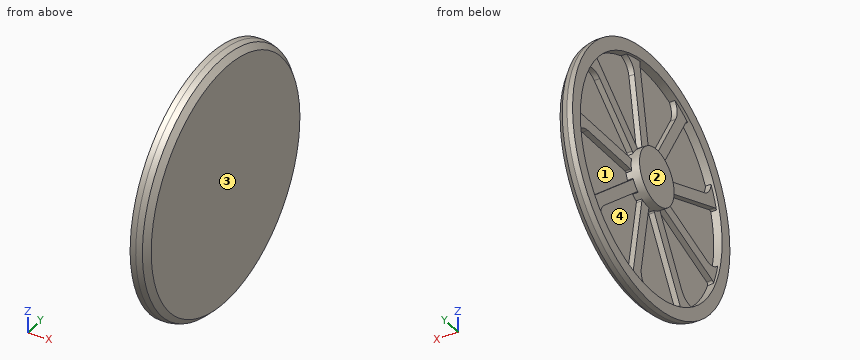
```python
from build123d import *

# Parameters (mm, degrees)
BOSS_EXTRU_1_DEPTH           = 20
R_P_TITION_CIRCULAIRE1_COUNT = 9


with BuildPart() as part:
    # Esquisse1 → Révolution1 (revolve)
    with BuildSketch(Plane.XY, mode=Mode.PRIVATE) as r_volution1_sk:
        Polygon((0, 0), (0, 430), (-19.509618943, 449.509618943), (-40, 455), (-60, 455), (-60, 410), (-30, 410), (-30, 100), (-80, 100), (-80, 0), align=None)
    revolve(r_volution1_sk.sketch.rotate(Axis((-80, 0, 0), (1, 0, 0)), 90), axis=Axis((-80, 0, 0), (1, 0, 0)))

    # Esquisse2 → Boss.-Extru.1 (add)
    with BuildSketch(Plane.ZY.offset(30)):
        with BuildLine():
            Line((-20, 104.612235173), (-20, 350.590090575))
            ThreePointArc((-20, 350.590090575), (-30.106477192, 383.916302208), (-57.021212726, 406.015493915))
            ThreePointArc((-57.021212726, 406.015493915), (-15.546179109, 409.705157784), (26.089198597, 409.169101615))
            ThreePointArc((26.089198597, 409.169101615), (21.660095503, 405.483324106), (20, 399.965535329))
            Line((20, 399.965535329), (20, 103.482062221))
            ThreePointArc((20, 103.482062221), (20.497231695, 100.367998231), (21.939478907, 97.563616504))
            ThreePointArc((21.939478907, 97.563616504), (-0.653338085, 99.997865724), (-23.212419248, 97.268615661))
            ThreePointArc((-23.212419248, 97.268615661), (-20.838236864, 100.60448066), (-20, 104.612235173))
        make_face()
    boss_extru_1 = extrude(amount=BOSS_EXTRU_1_DEPTH)

    # Répétition circulaire1: Boss.-Extru.1 ×9 about axis
    r_p_tition_circulaire1_axis = Axis((0, 0, 0), (1, 0, 0))
    for i in range(1, R_P_TITION_CIRCULAIRE1_COUNT):
        add(boss_extru_1.rotate(r_p_tition_circulaire1_axis, i * 360 / R_P_TITION_CIRCULAIRE1_COUNT))


solid = part.part
```
Verification items for the finished model (mm, model axes). Face numbers are marked on the shaded views. A direction names the side the tool comes from. Coordinates: 2 decimals unless noted, no trailing zeros. Write each loop counter-clockwise with the first axis right and the second up, starting at its lowest first coordinate (ties: lowest second). Pieces come first, ordered by that corner, then holes. Notation, with made-up numbers: M 45.25,41 L 87.25,41 A16 cw 87.25,71 Z; hole C 61,35 d4. An arc over 180 degrees is marked long. One line per item, written item: value.
Item 1: Mould release check, pull along Y, two halves, no side actions. Record for the marked faces 1 and 2: pulls with the +Y half, pulls with the -Y half, needs draft (parallel to the pull), parting line crosses it, or undercut.
Check sheet entries:
face 1: undercut
face 2: needs draft
Item 2: Section check A-A, the plane z = 0. Record the boundary of the cut face in (x, y).
Check sheet entries:
outline: M -80,-100 L -30,-100 L -30,-410 L -60,-410 L -60,-455 L -40,-455 L -19.51,-449.51 L 0,-430 L 0,430 L -19.51,449.51 L -40,455 L -60,455 L -60,410 L -50,410 L -50,100 L -80,100 Z
Item 3: Access from +Z, -Z, +X, -X, +Y, -Y to the whole of each face (thin tool, end or side, straight path). Record for the marked faces 3 and 4.
Check sheet entries:
face 3: +Z, -Z, +X, +Y, -Y
face 4: -X
Item 4: Gauge pin test, flat ends, axial feed: pin 1 Ø8 at (x, z) = (-63.5, -209.5) entering from +Y; pin 2 Ø10 at (x, z) = (-66.5, 97) entering from -Y; pin 3 Ø16 at (x, y) = (-41.5, 256.5) entering from -Z. Record the tip position at first contact, or that the pin passes through.
Check sheet entries:
pin 1: stops at y = 404.9
pin 2: stops at y = -39.19
pin 3: stops at z = -381.15
Item 5: Scan lines: line 1 along Y through (x, z) = (-52.75, 0); line 2 along Y through (x, z) = (-47, 0); line 3 along Z through (x, y) = (-31.5, -235). Record each from-to range of solid material in increasing order.
Check sheet entries:
line 1: y = -455 to -410, -100 to 100, 410 to 455
line 2: y = -455 to -410, -100 to 455
line 3: z = -386.95 to -322.85, -106.82 to -64.25, 64.25 to 106.82, 335.97 to 386.95
